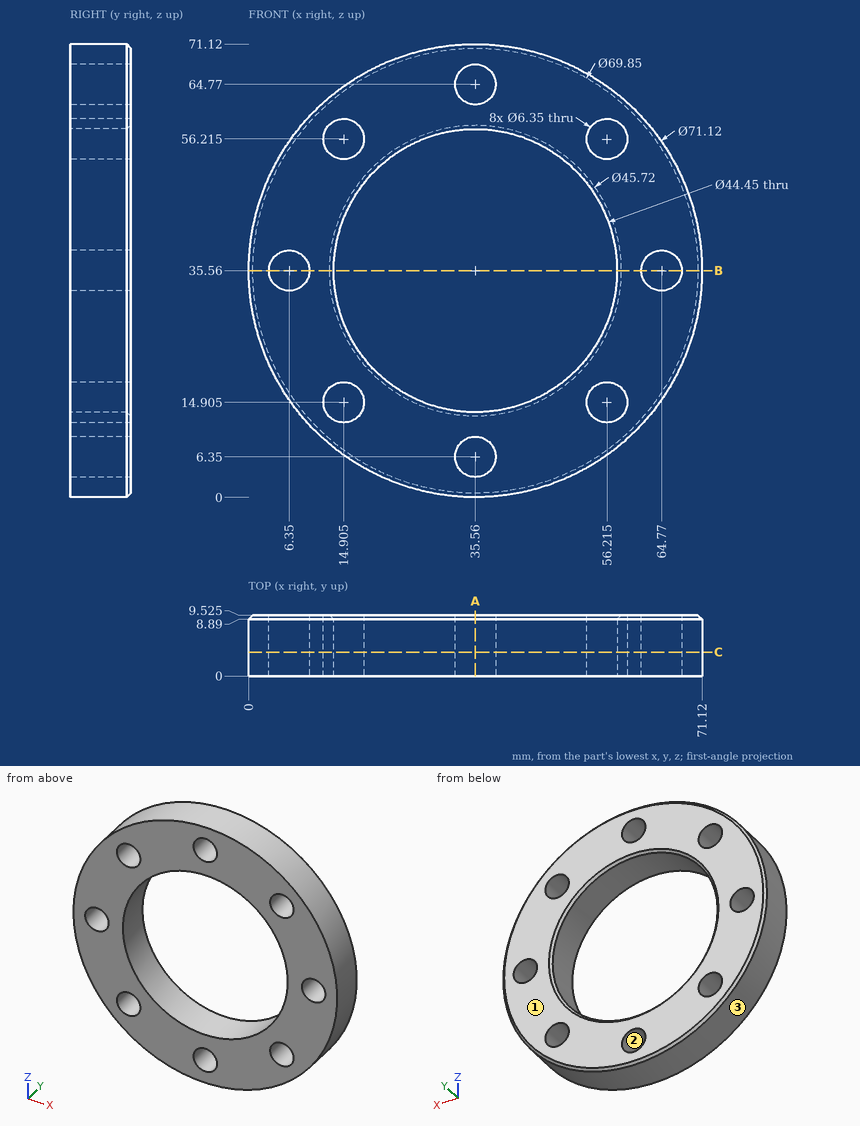
The drawing under review shows one solid part. Ordinate dimensions are in mm from its lowest x, y, z. Coordinates: 2 decimals unless noted, no trailing zeros. Write each loop counter-clockwise with the first axis right and the second up, starting at its lowest first coordinate (ties: lowest second). Pieces come first, ordered by that corner, then holes.
1) Add section B-B (z = 35.56). Write out the cut boundary in (x, y) (1 decimal), plus the area to 3 significant figures.
2) To check wall thickness, follow L1, parallel to X at y = 4.75, z = 58 (1 decimal); L2, parallel to X at y = 1.5, z = 37; L3, parallel to X at y = 6.5, z = 4 (1 decimal). State the ranges of each line that lie inside material, in increasing order.
3) Add section A-A (x = 35.56). Write out the cut boundary in (y, z) (1 decimal), plus the area to 3 significant figures.
4) Add section C-C (y = 3.75). State how many separate pieces and enclosed holes the cut face has, plus the area to 3 significant figures.
5) Mouldability with a two-part tool opening along X and no side actions: class the marked faces 1, 2 and 3 as +X half, -X half, draft (parallel to the pull), parting line (faces both ways), or undercut.
6) Insertion check: pin 1 (4 mm diameter, centred on y = 8, z = 56.5, fed in from +X); pin 2 (1.5 mm diameter, centred on y = 2, z = 13.5, fed in from -X); pin 3 (5 mm diameter, centred on x = 53.5, y = 3.5, fed in from +Z). Each pin has a flat end and moves straight along its axis. Give the tip position at first contact, or say it passes through.
Check result:
1. outline: (0, 0) - (3.2, 0) - (3.2, 9.5) - (0.6, 9.5) - (0, 8.9) - close; (9.5, 0) - (13.3, 0) - (13.3, 8.9) - (12.7, 9.5) - (9.5, 9.5) - close; (57.8, 0) - (61.6, 0) - (61.6, 9.5) - (58.4, 9.5) - (57.8, 8.9) - close; (67.9, 0) - (71.1, 0) - (71.1, 8.9) - (70.5, 9.5) - (67.9, 9.5) - close
1. area: 132 mm2
2. L1: x = 8 to 12.3, 17.5 to 53.6, 58.8 to 63.1
2. L2: x = 0.03 to 3.52, 9.18 to 13.38, 57.74 to 61.94, 67.6 to 71.09
2. L3: x = 19.2 to 33.4, 37.7 to 51.9
3. outline: (0, 0) - (8.9, 0) - (9.5, 0.6) - (9.5, 3.2) - (0, 3.2) - close; (0, 9.5) - (9.5, 9.5) - (9.5, 12.7) - (8.9, 13.3) - (0, 13.3) - close; (0, 57.8) - (8.9, 57.8) - (9.5, 58.4) - (9.5, 61.6) - (0, 61.6) - close; (0, 67.9) - (9.5, 67.9) - (9.5, 70.5) - (8.9, 71.1) - (0, 71.1) - close
3. area: 132 mm2
4. separate pieces: 1
4. enclosed holes: 9
4. area: 2,170 mm2
5. face 1: draft
5. face 2: undercut
5. face 3: parting line
6. pin 1: stops at x = 65.66
6. pin 2: stops at x = 7.09
6. pin 3: stops at z = 67.59
